from build123d import *

# Parameters (mm, degrees)
F2_R     = 1.75
F3_DEPTH = 12.5
F4_R     = 3
F5_R     = 2
F6_R     = 0.75


with BuildPart() as f1:
    # F0 (on Front) → F1 (revolve)
    with BuildSketch(Plane.XZ):
        Polygon((-9, 0), (0, 0), (0, 18), (-15, 18), (-15, 10), (-9, 8.721018), align=None)
    revolve(axis=Axis((0, 0, 9), (0, 0, 1)))

    # F2 (on face) → F3 (cut)
    with BuildSketch(Plane(origin=(0, 0, 0), x_dir=(1, 0, 0), z_dir=(0, 0, -1))):
        Circle(F2_R)
    extrude(amount=-F3_DEPTH, mode=Mode.SUBTRACT)

    # F4
    f4_edges = [f1.edges().sort_by_distance(p)[0] for p in [
        (15, 0, 18),
        (15, 0, 10),
    ]]
    fillet(f4_edges, radius=F4_R)

    # F5
    f5_edges = [f1.edges().sort_by_distance(p)[0] for p in [
        (9, 0, 8.721018),
    ]]
    fillet(f5_edges, radius=F5_R)

    # F6
    f6_edges = [f1.edges().sort_by_distance(p)[0] for p in [
        (9, 0, 0),
    ]]
    fillet(f6_edges, radius=F6_R)


solid = f1.part
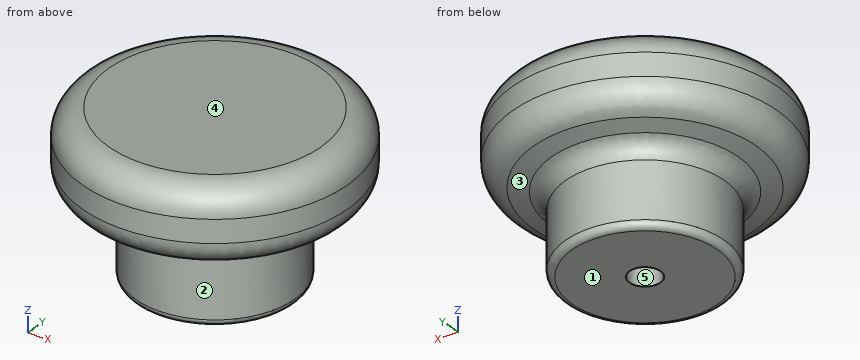
Read the model definition and answer for the solid it produces. Units are mm, in the model's axes. Face numbers are marked on the shaded views. A direction names the side the tool comes from. Round coordinates to 2 decimals unless told otherwise and drop trailing zeros. Write each loop counter-clockwise with the first axis right and the second up, starting at its lowest first coordinate (ties: lowest second). Pieces come first, ordered by that corner, then holes. Notation, with made-up numbers: (55.5, 54.5) - (69.5, 54.5) arc R28 ccw to (69.5, 79.5) - close; hole circle Ø4 at (-23.5, 10). An arc over 180 degrees is marked (long way). Use a Markdown table: item, result.
(1) Each of these flat-tipped pins is pushed along its axis until it touches: pin 1 Ø1.8 at (x, y) = (0, 0) entering from -Z; pin 2 Ø1.5 at (y, z) = (7.5, 4.5) entering from -X; pin 3 Ø2 at (y, z) = (7, 14.5) entering from +X. Where does it stop, or does it pass through?
Reported:
| item | result |
|---|---|
| pin 1 | z = 12.5 |
| pin 2 | x = -5.95 |
| pin 3 | x = 13.75 |
(2) The mould has two halves that part along Z. Classify the marked faces 3, 4 and 5: released by +Z, released by -Z, zero draft, split by the parting line, or undercut.
Reported:
| item | result |
|---|---|
| face 3 | released by -Z |
| face 4 | released by +Z |
| face 5 | zero draft |
(3) The part is cut by section A-A (z = 5.5). Write down the section's boundary in (x, y), then the cut area to 3 significant figures.
Reported:
| item | result |
|---|---|
| outline | circle Ø18 at (0, 0); hole circle Ø3.5 at (0, 0) |
| area | 245 mm2 |
(4) Straight lines are drawn through the part: line 1 along Y through (x, z) = (0, 4.75); line 2 along Y through (x, z) = (0, 8.5). For each, find the intervals that lie inside material, in ascending order. Write a range as [from, to].
Reported:
| item | result |
|---|---|
| line 1 | [-9, -1.75], [1.75, 9] |
| line 2 | [-9.57, -1.75], [1.75, 9.57] |
(5) Which of the six approach directions +Z, -Z, +X, -X, +Y, -Y give full straight-line access (tool end or side, diameter ignored) to the marked faces 1 and 2?
Reported:
| item | result |
|---|---|
| face 1 | -Z, +X, -X, +Y, -Y |
| face 2 | -Z |
